from build123d import *
from OCP.BRepFilletAPI import BRepFilletAPI_MakeChamfer

# Parameters (mm, degrees)
FILLET_1_R       = 2
FILLET_2_R       = 0.5
EXTRUDE_1_DEPTH  = 52
EXTRUDE_2_DEPTH  = 6
FILLET_3_R       = 1
CHAMFER_1_SIZE   = 6
CHAMFER_1_SIZE_2 = 0.5


with BuildPart() as part:
    # 스케치1 → 회전1 (revolve)
    with BuildSketch(Plane.XY, mode=Mode.PRIVATE) as revolve_1_sk:
        Polygon((0, 0), (51, 0), (51, 20), (50, 20), (49, 59), (50, 59), (50, 74), (0, 74), align=None)
    revolve(revolve_1_sk.sketch.rotate(Axis((0, 0, 0), (0, 1, 0)), 90), axis=Axis((0, 0, 0), (0, 1, 0)))

    # 필렛1
    fillet_1_edges = [part.edges().sort_by_distance(p)[0] for p in [
        (0, 74, 50),
        (0, 0, 51),
    ]]
    fillet(fillet_1_edges, radius=FILLET_1_R)

    # 필렛2
    fillet_2_edges = [part.edges().sort_by_distance(p)[0] for p in [
        (0, 59, 50),
        (0, 20, 51),
    ]]
    fillet(fillet_2_edges, radius=FILLET_2_R)

    # 스케치2 → 보스-돌출1 (add)
    with BuildSketch(Plane.XY):
        Polygon((0, 6.917096231), (3.5, 8.937822174), (3.5, 12.979274058), (0, 15), (-3.5, 12.979274058), (-3.5, 8.937822174), align=None)
    extrude(amount=EXTRUDE_1_DEPTH)

    # 스케치3 → 보스-돌출2 (add)
    with BuildSketch(Plane.XY.offset(52)):
        Polygon((-4, 8.649147039), (0, 6.339745962), (4, 8.649147039), (4, 13.267949192), (0, 15.577350269), (-4, 13.267949192), align=None)
    extrude(amount=EXTRUDE_2_DEPTH)

    # 필렛3
    fillet_3_edges = [part.edges().sort_by_distance(p)[0] for p in [
        (-4, 13.267949192, 55),
        (-4, 8.649147039, 55),
        (0, 6.339745962, 55),
        (4, 8.649147039, 55),
        (4, 13.267949192, 55),
        (0, 15.577350269, 55),
    ]]
    fillet(fillet_3_edges, radius=FILLET_3_R)

    # 모따기1
    chamfer_1_edges_1 = [part.edges().sort_by_distance(p)[0] for p in [
        (-2, 7.494446501, 58),
    ]]
    chamfer_1_side_1 = [part.faces().sort_by_distance(p)[0] for p in [
        (-2, 7.494446501, 57.99),
    ]]
    chamfer_1_edges_2 = [part.edges().sort_by_distance(p)[0] for p in [
        (0, 6.494446501, 58),
    ]]
    chamfer_1_side_2 = [part.faces().sort_by_distance(p)[0] for p in [
        (0, 6.494446501, 57.99),
    ]]
    chamfer_1_edges_3 = [part.edges().sort_by_distance(p)[0] for p in [
        (-3.866025404, 8.726497308, 58),
    ]]
    chamfer_1_side_3 = [part.faces().sort_by_distance(p)[0] for p in [
        (-3.866025404, 8.726497308, 57.99),
    ]]
    chamfer_1_edges_4 = [part.edges().sort_by_distance(p)[0] for p in [
        (2, 7.494446501, 58),
    ]]
    chamfer_1_side_4 = [part.faces().sort_by_distance(p)[0] for p in [
        (1.995, 7.503106755, 58),
    ]]
    chamfer_1_edges_5 = [part.edges().sort_by_distance(p)[0] for p in [
        (-4, 10.958548116, 58),
    ]]
    chamfer_1_side_5 = [part.faces().sort_by_distance(p)[0] for p in [
        (-3.99, 10.958548116, 58),
    ]]
    chamfer_1_edges_6 = [part.edges().sort_by_distance(p)[0] for p in [
        (3.866025404, 8.726497308, 58),
    ]]
    chamfer_1_side_6 = [part.faces().sort_by_distance(p)[0] for p in [
        (3.85736515, 8.731497308, 58),
    ]]
    chamfer_1_edges_7 = [part.edges().sort_by_distance(p)[0] for p in [
        (-3.866025404, 13.190598923, 58),
    ]]
    chamfer_1_side_7 = [part.faces().sort_by_distance(p)[0] for p in [
        (-3.85736515, 13.185598923, 58),
    ]]
    chamfer_1_edges_8 = [part.edges().sort_by_distance(p)[0] for p in [
        (4, 10.958548116, 58),
    ]]
    chamfer_1_side_8 = [part.faces().sort_by_distance(p)[0] for p in [
        (3.99, 10.958548116, 58),
    ]]
    chamfer_1_edges_9 = [part.edges().sort_by_distance(p)[0] for p in [
        (-2, 14.422649731, 58),
    ]]
    chamfer_1_side_9 = [part.faces().sort_by_distance(p)[0] for p in [
        (-1.995, 14.413989477, 58),
    ]]
    chamfer_1_edges_10 = [part.edges().sort_by_distance(p)[0] for p in [
        (3.866025404, 13.190598923, 58),
    ]]
    chamfer_1_side_10 = [part.faces().sort_by_distance(p)[0] for p in [
        (3.85736515, 13.185598923, 58),
    ]]
    chamfer_1_edges_11 = [part.edges().sort_by_distance(p)[0] for p in [
        (0, 15.422649731, 58),
    ]]
    chamfer_1_side_11 = [part.faces().sort_by_distance(p)[0] for p in [
        (0, 15.412649731, 58),
    ]]
    chamfer_1_edges_12 = [part.edges().sort_by_distance(p)[0] for p in [
        (2, 14.422649731, 58),
    ]]
    chamfer_1_side_12 = [part.faces().sort_by_distance(p)[0] for p in [
        (1.995, 14.413989477, 58),
    ]]
    chamfer_1 = BRepFilletAPI_MakeChamfer(part.part.solid().wrapped)
    for e in chamfer_1_edges_1:
        chamfer_1.Add(CHAMFER_1_SIZE - 0.0001, CHAMFER_1_SIZE_2 - 0.0001, e.wrapped, chamfer_1_side_1[0].wrapped)
    for e in chamfer_1_edges_2:
        chamfer_1.Add(CHAMFER_1_SIZE - 0.0001, CHAMFER_1_SIZE_2 - 0.0001, e.wrapped, chamfer_1_side_2[0].wrapped)
    for e in chamfer_1_edges_3:
        chamfer_1.Add(CHAMFER_1_SIZE - 0.0001, CHAMFER_1_SIZE_2 - 0.0001, e.wrapped, chamfer_1_side_3[0].wrapped)
    for e in chamfer_1_edges_4:
        chamfer_1.Add(CHAMFER_1_SIZE_2 - 0.0001, CHAMFER_1_SIZE - 0.0001, e.wrapped, chamfer_1_side_4[0].wrapped)
    for e in chamfer_1_edges_5:
        chamfer_1.Add(CHAMFER_1_SIZE_2 - 0.0001, CHAMFER_1_SIZE - 0.0001, e.wrapped, chamfer_1_side_5[0].wrapped)
    for e in chamfer_1_edges_6:
        chamfer_1.Add(CHAMFER_1_SIZE_2 - 0.0001, CHAMFER_1_SIZE - 0.0001, e.wrapped, chamfer_1_side_6[0].wrapped)
    for e in chamfer_1_edges_7:
        chamfer_1.Add(CHAMFER_1_SIZE_2 - 0.0001, CHAMFER_1_SIZE - 0.0001, e.wrapped, chamfer_1_side_7[0].wrapped)
    for e in chamfer_1_edges_8:
        chamfer_1.Add(CHAMFER_1_SIZE_2 - 0.0001, CHAMFER_1_SIZE - 0.0001, e.wrapped, chamfer_1_side_8[0].wrapped)
    for e in chamfer_1_edges_9:
        chamfer_1.Add(CHAMFER_1_SIZE_2 - 0.0001, CHAMFER_1_SIZE - 0.0001, e.wrapped, chamfer_1_side_9[0].wrapped)
    for e in chamfer_1_edges_10:
        chamfer_1.Add(CHAMFER_1_SIZE_2 - 0.0001, CHAMFER_1_SIZE - 0.0001, e.wrapped, chamfer_1_side_10[0].wrapped)
    for e in chamfer_1_edges_11:
        chamfer_1.Add(CHAMFER_1_SIZE_2 - 0.0001, CHAMFER_1_SIZE - 0.0001, e.wrapped, chamfer_1_side_11[0].wrapped)
    for e in chamfer_1_edges_12:
        chamfer_1.Add(CHAMFER_1_SIZE_2 - 0.0001, CHAMFER_1_SIZE - 0.0001, e.wrapped, chamfer_1_side_12[0].wrapped)
    add(Compound.cast(chamfer_1.Shape()), mode=Mode.REPLACE)  # a hair under: the kernel refuses the full size


solid = part.part
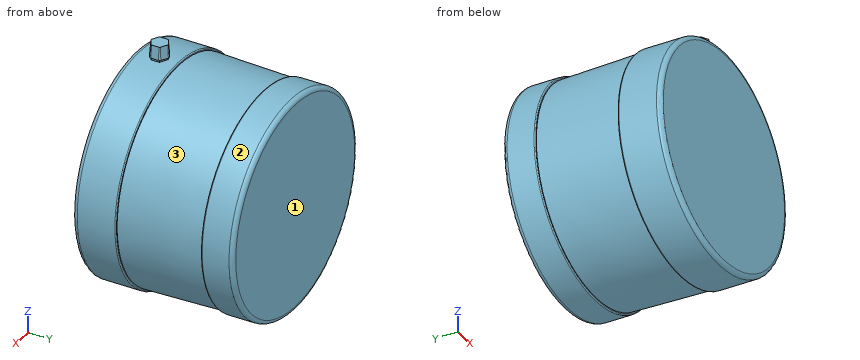
Build history of the part. All positions in model axes, mm. Face numbers are marked on the shaded views. A direction names the side the tool comes from. Give positions to 0.01 mm unless a question says otherwise; leave off trailing zeros. Order: outer loops, then holes, each group sorted by start corner. A loop starts at its lowest first (then second) coordinate and runs counter-clockwise, first axis right, second up. Notation, with made-up numbers: M 19.25,-28 L 64.25,-28 A32 ccw 64.25,0 Z; hole C 49,75.5 d9. An arc over 180 degrees is marked long. Put each result on its own line as item: value.
Item 1: Slice it at A-A, the plane z = 0. Write the cut outline in (x, y).
From the geometry:
outline: M -51,2 A2 ccw -49,0 L 49,0 A2 ccw 51,2 L 51,19.5 A0.5 ccw 50.5,20 L 50,20 L 49,59 L 49.5,59 A0.5 ccw 50,59.5 L 50,72 A2 ccw 48,74 L -48,74 A2 ccw -50,72 L -50,59.5 A0.5 ccw -49.5,59 L -49,59 L -50,20 L -50.5,20 A0.5 ccw -51,19.5 Z
Item 2: Flat gauge pins, fed straight in: pin 1 Ø1.5 at (y, z) = (27, -21.5) entering from +X; pin 2 Ø1 at (x, y) = (36, 51) entering from -Z; pin 3 Ø2 at (y, z) = (46, -20.5) entering from -X. Where does each tip first touch, or does it go through?
From the geometry:
pin 1: stops at x = 45.29
pin 2: stops at z = -34.07
pin 3: stops at x = -45.32
Item 3: Probe line 1 (X direction, y = 51.5, z = -42); line 2 (Z direction, x = 23, y = 27); line 3 (Z direction, x = -9.5, y = 30). List the from-to ranges inside material, lowest first. Write a range as [from, to].
From the geometry:
line 1: x = [-25.61, 25.61]
line 2: z = [-44.19, 44.19]
line 3: z = [-48.83, 48.83]
Item 4: Slice it at C-C, the plane y = 5. Write the cut outline in (x, z), plus the area to 3 significant figures.
From the geometry:
outline: C 0,0 d102
area: 8,170 mm2
Item 5: Slice it at B-B, the plane y = 63.5. Write the cut outline in (x, z), plus the area to 3 significant figures.
From the geometry:
outline: C 0,0 d100
area: 7,850 mm2
Item 6: 3-axis set-ups, long thin cutter, end or side, ignore diameter. For the marked faces 1, 2 and 3: which of +Z, -Z, +X, -X, +Y, -Y reach the whole face in a straight line?
From the geometry:
face 1: +Z, -Z, +X, -X, +Y
face 2: +Y
face 3: none
